The drawing under review shows one solid part. Ordinate dimensions are in mm from its lowest x, y, z. A direction names the side the tool comes from. Give positions to 0.01 mm unless a question says otherwise; leave off trailing zeros. Order: outer loops, then holes, each group sorted by start corner. A loop starts at its lowest first (then second) coordinate and runs counter-clockwise, first axis right, second up. Notation, with made-up numbers: (87, -14) - (92, -14) arc R21 cw to (92, -10) - close; hole circle Ø10 at (23, 38). An arc over 180 degrees is marked (long way). Use CSV: the item, a comma, the result in double quotes.
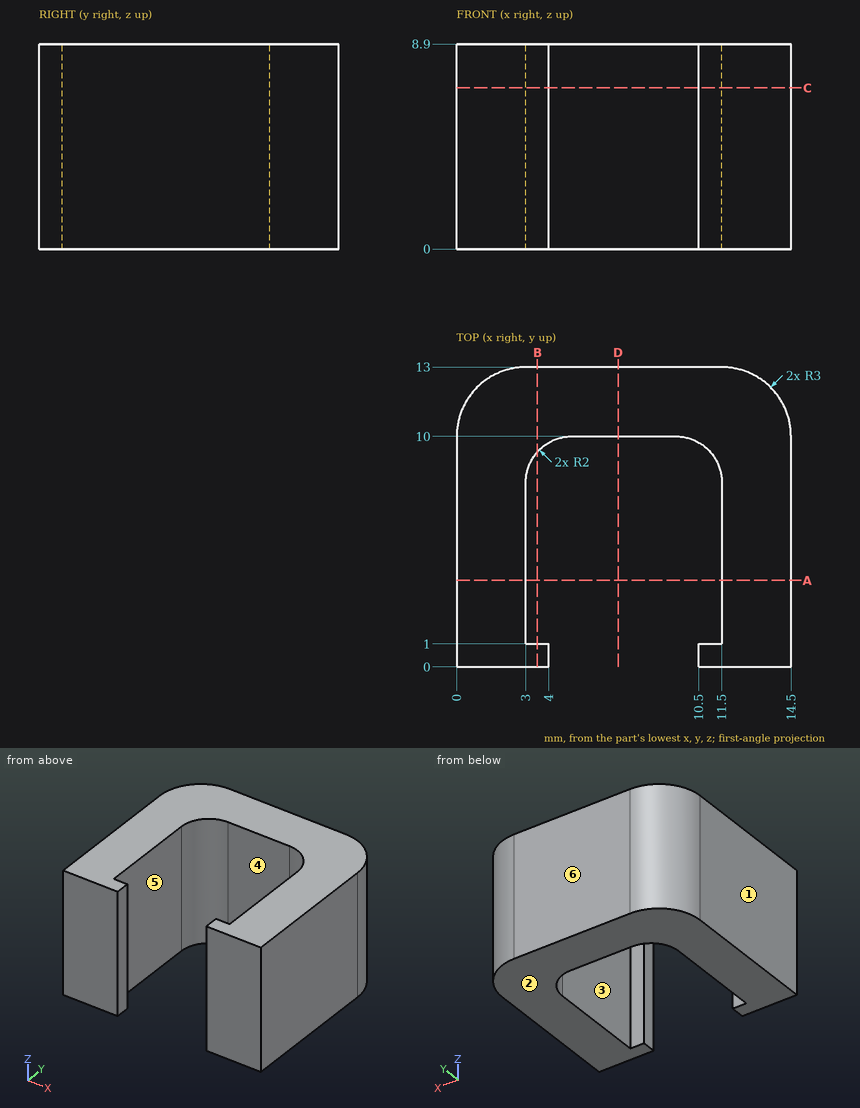
Item 1: Take a section at D-D, the plane x = 7. Give the boundary of the cut face in (y, z).
Results list:
outline,"(10, 0) - (13, 0) - (13, 8.9) - (10, 8.9) - close"
Item 2: Take a section at A-A, the plane y = 3.75. Give the boundary of the cut face in (x, z), and give its area (3 significant figures).
Results list:
outline,"(0, 0) - (3, 0) - (3, 8.9) - (0, 8.9) - close; (11.5, 0) - (14.5, 0) - (14.5, 8.9) - (11.5, 8.9) - close"
area,"53.4 mm2"
Item 3: Take a section at C-C, the plane z = 7. Give the boundary of the cut face in (x, y).
Results list:
outline,"(0, 0) - (4, 0) - (4, 1) - (3, 1) - (3, 8) arc R2 cw to (5, 10) - (9.5, 10) arc R2 cw to (11.5, 8) - (11.5, 1) - (10.5, 1) - (10.5, 0) - (14.5, 0) - (14.5, 10) arc R3 ccw to (11.5, 13) - (3, 13) arc R3 ccw to (0, 10) - close"
Item 4: Wall thickness on L1, parallel to X at y = 5.5, z = 3.5; L2, parallel to Y at x = 6.75, z = 7.75; L3, parallel to Y at x = 10.75, z = 3.75: over which ranges is each line inside the solid? List them lowest first.
Results list:
L1,"x = 0 to 3, 11.5 to 14.5"
L2,"y = 10 to 13"
L3,"y = 0 to 1, 9.56 to 13"
Item 5: Mouldability with a two-part tool opening along X and no side actions: class the marked faces 1, 2 and 3 as pulls with the +X half, pulls with the -X half, needs draft (parallel to the pull), parting line crosses it, or undercut.
Results list:
face 1,"pulls with the -X half"
face 2,"needs draft"
face 3,"undercut"
Item 6: Tool access review of the marked faces 4, 5 and 6: name each direction out of +Z, -Z, +X, -X, +Y, -Y from which nothing blocks a thin tool from reaching the whole face with its end or side.
Results list:
face 4,"+Z, -Z, -Y"
face 5,"+Z, -Z"
face 6,"+Z, -Z, +X, -X, +Y"
Item 7: Take a section at B-B, the plane x = 3.5. Give the boundary of the cut face in (y, z), and give its area (3 significant figures).
Results list:
outline,"(0, 0) - (1, 0) - (1, 8.9) - (0, 8.9) - close; (9.32, 0) - (13, 0) - (13, 8.9) - (9.32, 8.9) - close"
area,"41.6 mm2"
